Read the model definition and answer for the solid it produces. Units are mm, in the model's axes. A direction names the side the tool comes from. Coordinates: 2 decimals unless noted, no trailing zeros. Order: outer loops, then holes, each group sorted by start corner. A loop starts at its lowest first (then second) coordinate and runs counter-clockwise, first axis right, second up.
```python
from build123d import *

# Parameters (mm, degrees)
BOSS_EXTRUDE1_DEPTH = 3.175
SKETCH2_W           = 12.7
SKETCH2_H           = 6.35
CUT_EXTRUDE1_DEPTH  = 3.175
FILLET1_R           = 7.62
FILLET2_R           = 2.54
SKETCH3_W           = 71.12
SKETCH3_H           = 3.175
BOSS_EXTRUDE2_DEPTH = 4.7625


with BuildPart() as part:
    # Sketch1 → Boss-Extrude1 (new body)
    with BuildSketch(Plane(origin=(0, 0, 0), x_dir=(1, 0, 0), z_dir=(0, 1, 0))):
        Polygon((0, 0), (-147.828, 0), (-27.432, 303.022), (0, 303.022), align=None)
    extrude(amount=BOSS_EXTRUDE1_DEPTH)

    # Sketch2 → Cut-Extrude1 (cut)
    with BuildSketch(Plane(origin=(0, 3.175, 0), x_dir=(1, 0, 0), z_dir=(0, 1, 0))):
        with Locations((-13.716, 299.847)):
            Rectangle(SKETCH2_W, SKETCH2_H)
        Polygon((-25.4, 25.4), (-25.4, 239.346487548), (-110.404723468, 25.4), align=None)
    extrude(amount=-CUT_EXTRUDE1_DEPTH, mode=Mode.SUBTRACT)

    # Fillet1
    fillet1_edges = [part.edges().sort_by_distance(p)[0] for p in [
        (-25.4, 1.5875, -25.4),
        (-110.404723468, 1.5875, -25.4),
    ]]
    fillet(fillet1_edges, radius=FILLET1_R)

    # Fillet2
    fillet2_edges = [part.edges().sort_by_distance(p)[0] for p in [
        (-25.4, 1.5875, -239.346487548),
    ]]
    fillet(fillet2_edges, radius=FILLET2_R)

    # Sketch3 → Boss-Extrude2 (add)
    with BuildSketch(Plane.XY):
        with Locations((-73.914, 1.5875)):
            Rectangle(SKETCH3_W, SKETCH3_H)
    extrude(amount=BOSS_EXTRUDE2_DEPTH)


solid = part.part
```
1) Determine the mould class of faces 3 (the flat face through (-88.473, 1.565, -149.39)), 4 (the flat face through (-24, 3.175, -117)), 5 (the flat face through (-67.75, 1.61, -132.76)) for opening direction Z: pulls with the +Z half, pulls with the -Z half, needs draft (parallel to the pull), parting line crosses it, or undercut.
A:
face 3: pulls with the -Z half
face 4: needs draft
face 5: undercut
2) Flat-ended cylindrical pins translate along their axes: pin 1 Ø1.6 at (x, y) = (-129.5, 1.5) entering from +Z; pin 2 Ø1.6 at (y, z) = (2, 1.5) entering from +X; pin 3 Ø1.6 at (y, z) = (1, -125.5) entering from -X. Find the tip coordinate at first contact, or state that the pin passes through.
A:
pin 1: stops at z = 0
pin 2: stops at x = -38.35
pin 3: stops at x = -98.28
3) A cutting plane is placed at B-B, the plane y = 0.55. Determine the outline of the cut face in (x, z).
A:
outline: (-147.83, 0) - (-27.43, -303.02) - (-20.07, -303.02) - (-20.07, -296.67) - (-7.37, -296.67) - (-7.37, -303.02) - (0, -303.02) - (0, 0) - (-38.35, 0) - (-38.35, 4.76) - (-109.47, 4.76) - (-109.47, 0) - close; hole (-106.26, -35.83) - (-30.3, -227.01) arc R2.54 ccw to (-25.4, -226.07) - (-25.4, -33.02) arc R7.62 ccw to (-33.02, -25.4) - (-99.18, -25.4) arc R7.62 ccw to start
4) A cutting plane is placed at D-D, the plane x = -17. Determine the outline of the cut face in (y, z) (3 decimals), and give its area (3 significant figures).
A:
outline: (0, -296.672) - (3.175, -296.672) - (3.175, 0) - (0, 0) - close
area: 942 mm2
5) A cutting plane is placed at A-A, the plane z = -196.5. Determine the outline of the cut face in (x, y) (3 decimals), and give its area (3 significant figures).
A:
outline: (-69.755, 0) - (-42.424, 0) - (-42.424, 3.175) - (-69.755, 3.175) - close; (-25.4, 0) - (0, 0) - (0, 3.175) - (-25.4, 3.175) - close
area: 167 mm2
6) Which of the six approach directions +Z, -Z, +X, -X, +Y, -Y give full straight-line access (tool end or side, diameter ignored) to faces 1 (the cylindrical face through (-105.424, 1.565, -28.655)), 2 (the flat face through (-24, 0, -117))?
A:
face 1: +Y, -Y
face 2: +Z, -Z, +X, -X, -Y
7) Straight lines are drawn through the part: line 1 (X direction, y = 1.85, z = -92); line 2 (X direction, y = 0.95, z = -115.5); line 3 (Z direction, x = -9, y = 2.25). For each, find the intervals that lie inside material, in ascending order.
A:
line 1: x = -111.27 to -83.94, -25.4 to 0
line 2: x = -101.94 to -74.61, -25.4 to 0
line 3: z = -296.67 to 0
8) A cutting plane is placed at C-C, the plane x = -84. Determine the outline of the cut face in (y, z) (1 decimal).
A:
outline: (0, -160.6) - (3.2, -160.6) - (3.2, -91.9) - (0, -91.9) - close; (0, -25.4) - (3.2, -25.4) - (3.2, 4.8) - (0, 4.8) - close
